Input: dimensioned drawing with shaded views. Units: mm. Origin: part minimum x, y, z. A direction names the side the tool comes from. Coordinates: 2 decimals unless noted, no trailing zeros. Write each loop counter-clockwise with the first axis right and the second up, starting at its lowest first coordinate (ties: lowest second). Pieces come first, ordered by that corner, then holes. Notation, with made-up numbers: (-6, 24) - (30, 24) arc R17 ccw to (30, 36) - close; hole circle Ø11 at (70, 45). An arc over 180 degrees is marked (long way). One line per question, with ' | ' between items.
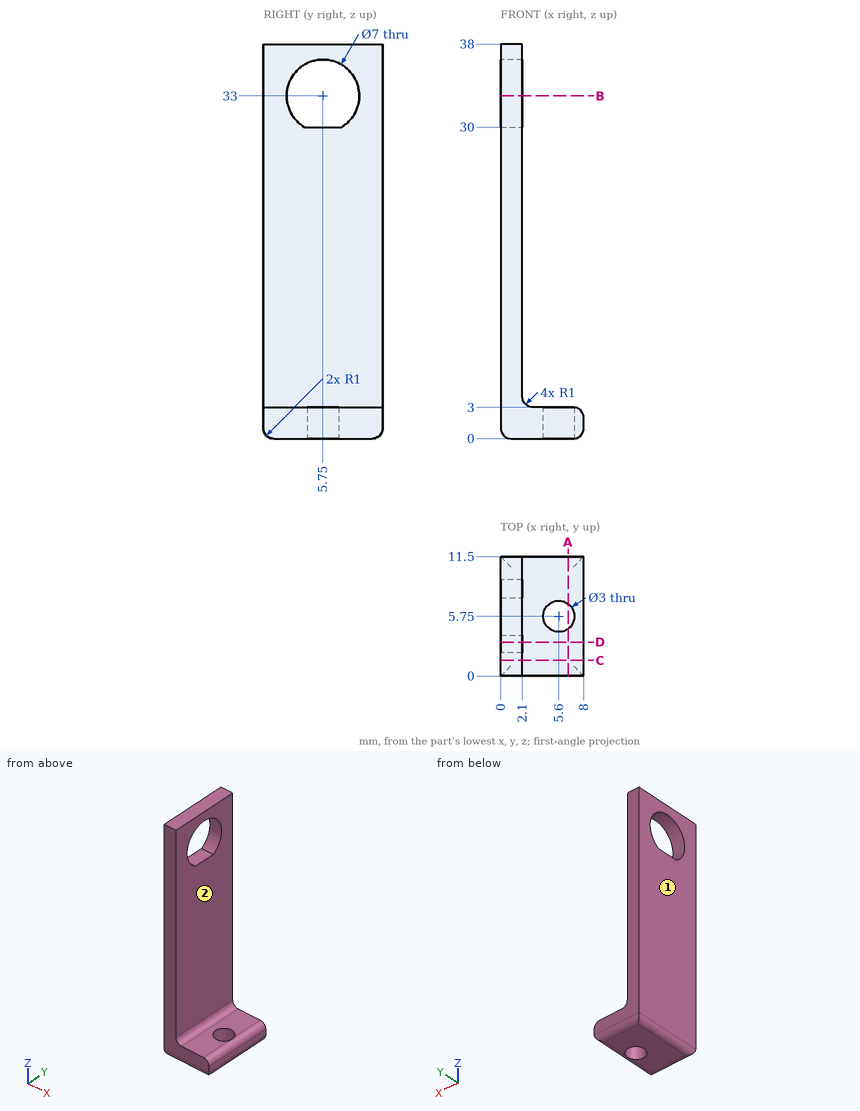
Item 1: Pin query (flat end, axial travel): pin 1 Ø1.2 at (x, y) = (6, 5.5) entering from +Z; pin 2 Ø3 at (x, z) = (2.5, 16) entering from -Y; pin 3 Ø6.5 at (y, z) = (5.75, 33) entering from +X; pin 4 Ø3 at (y, z) = (6, 5) entering from +X. Return the tip coordinate at first contact, or that it passes through.
Check sheet entries:
pin 1: through | pin 2: y = 0 | pin 3: x = 2.1 | pin 4: x = 2.23
Item 2: Cut plane B-B on z = 33. Return loops of the section in (x, y).
Check sheet entries:
outline: (0, 0) - (2.1, 0) - (2.1, 2.25) - (0, 2.25) - close; (0, 9.25) - (2.1, 9.25) - (2.1, 11.5) - (0, 11.5) - close
Item 3: Cut plane A-A on x = 6.5. Return loops of the section in (y, z).
Check sheet entries:
outline: (0, 1) arc R1 ccw to (1, 0) - (4.55, 0) - (4.55, 3) - (0, 3) - close; (6.95, 0) - (10.5, 0) arc R1 ccw to (11.5, 1) - (11.5, 3) - (6.95, 3) - close
Item 4: Access query for the marked faces 1 and 2. Directions: +Z, -Z, +X, -X, +Y, -Y. A direction counts if a zero-diameter tool reaches every point of the face in a straight line with its end or side. Return the directions, or none.
Check sheet entries:
face 1: +Z, -Z, -X, +Y, -Y | face 2: +Z, +X, +Y, -Y
Item 5: Cut plane D-D on y = 3.25. Return loops of the section in (x, z), and give its area (3 significant figures).
Check sheet entries:
outline: (0, 1) arc R1 ccw to (1, 0) - (7, 0) arc R1 ccw to (8, 1) - (8, 2) arc R1 ccw to (7, 3) - (3.1, 3) arc R1 cw to (2.1, 4) - (2.1, 30.55) - (0, 30.55) - close; (0, 35.45) - (2.1, 35.45) - (2.1, 38) - (0, 38) - close | area: 86.8 mm²
Item 6: Ray query, line 1 along Y through (x, z) = (1.4, 33); line 2 along Y through (x, z) = (5.6, 0.95); line 3 along X through (y, z) = (5.5, 26.5). Return the intervals inside material, ascending. Write a range as [from, to].
Check sheet entries:
line 1: [0, 2.25], [9.25, 11.5] | line 2: [0, 4.25], [7.25, 11.5] | line 3: [0, 2.1]
Item 7: Cut plane C-C on y = 1.5. Return loops of the section in (x, z), and give its area (3 significant figures).
Check sheet entries:
outline: (0, 1) arc R1 ccw to (1, 0) - (7, 0) arc R1 ccw to (8, 1) - (8, 2) arc R1 ccw to (7, 3) - (3.1, 3) arc R1 cw to (2.1, 4) - (2.1, 38) - (0, 38) - close | area: 97.1 mm²
